```python
from build123d import *

# Parameters (mm, degrees)
BOSS_EXTRUDE1_DEPTH              = 20
SKETCH8_W                        = 42
SKETCH8_H                        = 60
CUT_EXTRUDE1_DEPTH               = 15
CUT_EXTRUDE2_START               = -5
CUT_EXTRUDE2_DEPTH               = 5
SKETCH10_R                       = 36
CUT_EXTRUDE3_DEPTH               = 157.424129235
SKETCH11_R                       = 41
SKETCH11_R_2                     = 36
BOSS_EXTRUDE4_DEPTH              = 5
SKETCH13_W                       = 106.111938503
SKETCH13_H                       = 55
SKETCH13_R                       = 3
BOSS_EXTRUDE9_DEPTH              = 20
BOSS_EXTRUDE13_START             = -5
SKETCH14_R                       = 36
SKETCH14_R_2                     = 33.5
BOSS_EXTRUDE13_DEPTH             = 5
FILLET1_R                        = 10
CUT_EXTRUDE4_DEPTH               = 6
CBORE_FOR_M6_5_SHSS1_D           = 7.1
CBORE_FOR_M6_5_SHSS1_CBORE_D     = 11
CBORE_FOR_M6_5_SHSS1_CBORE_DEPTH = 4.5
CHAMFER5_SIZE                    = 10.579618843
CHAMFER5_SIZE_2                  = 60
CUT_EXTRUDE5_DEPTH               = 1
SKETCH23_W                       = 20
SKETCH23_H                       = 8
CUT_EXTRUDE6_DEPTH               = 34
FILLET5_R                        = 2


with BuildPart() as part:
    # Sketch1 → Boss-Extrude1 (new body)
    with BuildSketch(Plane(origin=(0, 0, 0), x_dir=(1, 0, 0), z_dir=(0, 1, 0))):
        with BuildLine():
            Line((48.082138056, 60.239377577), (47.498980657, -45.87095849))
            ThreePointArc((47.498980657, -45.87095849), (-20.370958489, -112.998980658), (-87.498980658, -45.129041511))
            Line((-87.498980658, -45.129041511), (-86.915823259, 60.981294555))
            ThreePointArc((-86.915823259, 60.981294555), (-19.045884112, 128.109316723), (48.082138056, 60.239377577))
        make_face()
    extrude(amount=BOSS_EXTRUDE1_DEPTH)

    # Sketch8 → Cut-Extrude1 (cut)
    with BuildSketch(Plane.XZ):
        with Locations((-20, -62.5)):
            Rectangle(SKETCH8_W, SKETCH8_H)
    extrude(amount=-CUT_EXTRUDE1_DEPTH, mode=Mode.SUBTRACT)

    # Cut-Extrude2: read off the stored shape, not the designer's step
    # Cut-Extrude2 outline → Cut-Extrude2 (cut)
    with BuildSketch(Plane.XZ.offset(-15).offset(CUT_EXTRUDE2_START)):
        with BuildLine():
            Line((-6.5, -34.5), (-6.5, -90.5))
            ThreePointArc((-6.5, -90.5), (-4.5, -92.5), (-2.5, -90.5))
            Line((-2.5, -90.5), (-2.5, -34.5))
            ThreePointArc((-2.5, -34.5), (-4.5, -32.5), (-6.5, -34.5))
        make_face()
        with BuildLine():
            ThreePointArc((-8, -45), (-20, -33), (-32, -45))
            Line((-32, -45), (-32, -80))
            ThreePointArc((-32, -80), (-20, -92), (-8, -80))
            Line((-8, -80), (-8, -45))
        make_face()
        with BuildLine():
            Line((-37.5, -34.5), (-37.5, -90.5))
            ThreePointArc((-37.5, -90.5), (-35.5, -92.5), (-33.5, -90.5))
            Line((-33.5, -90.5), (-33.5, -34.5))
            ThreePointArc((-33.5, -34.5), (-35.5, -32.5), (-37.5, -34.5))
        make_face()
    extrude(amount=CUT_EXTRUDE2_DEPTH, mode=Mode.SUBTRACT)

    # Sketch10 → Cut-Extrude3 (cut, through all)
    with BuildSketch(Plane.XZ):
        with Locations(Location((-20, 45.5, 0), (0, 0, 270))):
            Circle(SKETCH10_R)
    extrude(amount=-CUT_EXTRUDE3_DEPTH, mode=Mode.SUBTRACT)

    # Sketch11 → Boss-Extrude4 (add)
    with BuildSketch(Plane(origin=(0, 20, 0), x_dir=(1, 0, 0), z_dir=(0, 1, 0))):
        with Locations(Location((-20, -45.5, 0), (0, 0, 270))):
            Circle(SKETCH11_R)
        with Locations(Location((-20, -45.5, 0), (0, 0, 90))):
            Circle(SKETCH11_R_2, mode=Mode.SUBTRACT)
    extrude(amount=BOSS_EXTRUDE4_DEPTH)

    # Sketch13 → Boss-Extrude9 (add)
    with BuildSketch(Plane(origin=(27.749936459, 0, 0.152507111), x_dir=(-0.00549568132488102, 0, 0.999984898629362), z_dir=(-0.999984898629362, 0, -0.00549568132488102))):
        with Locations((-7.446742736, -27.5)):
            Rectangle(SKETCH13_W, SKETCH13_H)
        with Locations((-25.004242736, -10.014310552)):
            Circle(SKETCH13_R, mode=Mode.SUBTRACT)
        with Locations((10.110757264, -10.014310552)):
            Circle(SKETCH13_R, mode=Mode.SUBTRACT)
        with Locations((10.110757264, -39.577999726)):
            Circle(SKETCH13_R, mode=Mode.SUBTRACT)
        with Locations((-25.004242736, -39.514310552)):
            Circle(SKETCH13_R, mode=Mode.SUBTRACT)
    extrude(amount=-BOSS_EXTRUDE9_DEPTH)

    # Sketch14 → Boss-Extrude13 (add)
    with BuildSketch(Plane(origin=(0, 16, 0), x_dir=(1, 0, 0), z_dir=(0, 1, 0)).offset(BOSS_EXTRUDE13_START)):
        with Locations(Location((-20, -45.5, 0), (0, 0, 90))):
            Circle(SKETCH14_R)
        with Locations(Location((-20, -45.5, 0), (0, 0, 270))):
            Circle(SKETCH14_R_2, mode=Mode.SUBTRACT)
    extrude(amount=BOSS_EXTRUDE13_DEPTH)

    # Fillet1
    # the kernel refuses this fillet: 10 mm, written as the material it adds along each edge
    with BuildSketch(Plane(origin=(-20, 11, 45.5), x_dir=(0, 0, -1), z_dir=(1, 0, 0))) as fillet1_piece_1:
        with BuildLine():
            CenterArc((26, -6.614378278), FILLET1_R, 0, 41.409622109)
            Line((36, -6.614378278), (36.2, -6.614378278))
            Line((36.2, -6.614378278), (36.2, 0))
            Line((36.2, 0), (36, 0.2))
            ThreePointArc((36, 0.2), (34.75, 0.2), (33.65, 0.132287566))
            Line((33.65, 0.132287566), (33.5, 0))
        make_face()
    revolve(axis=Axis((-20, 11, 45.5), (0, 1, 0)))

    # Sketch15 → Cut-Extrude4 (cut)
    with BuildSketch(Plane.XZ):
        with BuildLine():
            Line((27.499282685, 45.761044864), (47.498980657, 45.87095849))
            ThreePointArc((47.498980657, 45.87095849), (-20.370958489, 112.998980658), (-87.498980658, 45.129041511))
            Line((-87.498980658, 45.129041511), (-86.915823259, -60.981294555))
            ThreePointArc((-86.915823259, -60.981294555), (-19.045884112, -128.109316723), (48.082138056, -60.239377577))
            Line((48.082138056, -60.239377577), (28.082440084, -60.349291203))
            Line((28.082440084, -60.349291203), (27.499282685, 45.761044864))
        make_face()
    extrude(amount=-CUT_EXTRUDE4_DEPTH, mode=Mode.SUBTRACT)

    # CBORE for M6.5 SHSS1 (through all)
    with Locations(Plane(origin=(27.749936459, 0, 0.152507111), x_dir=(-0.005495681324881029, 0, 0.999984898629362), z_dir=(-0.999984898629362, 0, -0.005495681324881029))):
        with Locations((10.110757264, -39.577999726), (-25.004242736, -39.514310552), (10.110757264, -10.014310552), (-25.004242736, -10.014310552)):
            CounterBoreHole(CBORE_FOR_M6_5_SHSS1_D / 2, CBORE_FOR_M6_5_SHSS1_CBORE_D / 2, CBORE_FOR_M6_5_SHSS1_CBORE_DEPTH)

    # Chamfer5
    # the kernel refuses this chamfer: 60, 10.579618843 mm, written as the material it adds along each edge
    with BuildSketch(Plane(origin=(28.939284552, 6, -216.259264498), x_dir=(-0.9999848986293619, 0, -0.00549568132488103), z_dir=(-0.00549568132488103, 0, 0.999984898629362))) as chamfer5_piece_1_section:
        Polygon((CHAMFER5_SIZE, 0), (0, CHAMFER5_SIZE_2), (0, 0), align=None)
    chamfer5_piece_1 = extrude(amount=417.936594073, mode=Mode.PRIVATE)
    chamfer5_piece_1 = chamfer5_piece_1 - Plane(origin=(27.887351809, -10.014310552, -24.851358027), x_dir=(-0.005495681324881029, 0, 0.999984898629362), z_dir=(-0.999984898629362, 0, -0.005495681324881029)) * Cylinder(5.5, 1076, mode=Mode.PRIVATE)
    chamfer5_piece_1 = chamfer5_piece_1 - Plane(origin=(27.694370959, -10.014310552, 10.263111688), x_dir=(-0.005495681324881029, 0, 0.999984898629362), z_dir=(-0.999984898629362, 0, -0.005495681324881029)) * Cylinder(5.5, 1076, mode=Mode.PRIVATE)
    chamfer5_piece_1 = chamfer5_piece_1 - Plane(origin=(27.887351809, -39.514310552, -24.851358027), x_dir=(-0.005495681324881029, 0, 0.999984898629362), z_dir=(-0.999984898629362, 0, -0.005495681324881029)) * Cylinder(5.5, 1076, mode=Mode.PRIVATE)
    chamfer5_piece_1 = chamfer5_piece_1 - Plane(origin=(27.694370959, -39.577999726, 10.263111688), x_dir=(-0.005495681324881029, 0, 0.999984898629362), z_dir=(-0.999984898629362, 0, -0.005495681324881029)) * Cylinder(5.5, 1076, mode=Mode.PRIVATE)
    chamfer5_piece_1 = split(chamfer5_piece_1, bisect_by=Plane(origin=(27.486315043, -40.618009932, 48.120615135), z_dir=(0.0054121895768273285, 0.17364817766693125, -0.9847928810653225)), keep=Keep.TOP, mode=Mode.PRIVATE)
    chamfer5_piece_1 = split(chamfer5_piece_1, bisect_by=Plane(origin=(28.164666117, 30.853356971, -75.311001495), z_dir=(-0.00541218957682626, 0.17364817766693136, 0.9847928810653225)), keep=Keep.TOP, mode=Mode.PRIVATE)
    add(chamfer5_piece_1)
    with BuildSketch(Plane(origin=(203.992111352, 6, -59.382533108), x_dir=(0.005495681324880034, 0, -0.9999848986293619), z_dir=(-0.999984898629362, 0, -0.005495681324880034))) as chamfer5_piece_2_section:
        Polygon((CHAMFER5_SIZE, 0), (0, CHAMFER5_SIZE_2), (0, 0), align=None)
    chamfer5_piece_2 = extrude(amount=331.824655571, mode=Mode.PRIVATE)
    chamfer5_piece_2 = chamfer5_piece_2 & Plane(origin=(-19.416842601, 6, -60.610336066), x_dir=(-0.999984898629362, 0, -0.005495681324881549), z_dir=(0, -1, 0)) * Cylinder(67.5, 904, mode=Mode.PRIVATE)
    chamfer5_piece_2 = split(chamfer5_piece_2, bisect_by=Plane(origin=(23.126316359, -25.892001157, -60.376528891), z_dir=(0.9847928810653225, 0.1736481776669314, 0.005412189576827241)), keep=Keep.TOP, mode=Mode.PRIVATE)
    add(chamfer5_piece_2)
    with BuildSketch(Plane(origin=(-128.410690611, 6, 44.904200396), x_dir=(-0.005495681324881117, 0, 0.9999848986293619), z_dir=(0.999984898629362, 0, 0.005495681324881118))) as chamfer5_piece_3_section:
        Polygon((CHAMFER5_SIZE, 0), (0, CHAMFER5_SIZE_2), (0, 0), align=None)
    chamfer5_piece_3 = extrude(amount=331.824655571, mode=Mode.PRIVATE)
    chamfer5_piece_3 = chamfer5_piece_3 & Plane(origin=(-20, 6, 45.500000001), x_dir=(0.999984898629362, 0, 0.0054956813248813385), z_dir=(0, -1, 0)) * Cylinder(67.5, 904, mode=Mode.PRIVATE)
    chamfer5_piece_3 = split(chamfer5_piece_3, bisect_by=Plane(origin=(12.537572393, 30.853356971, 45.67881883), z_dir=(0.9847928810653225, 0.1736481776669314, 0.005412189576827241)), keep=Keep.TOP, mode=Mode.PRIVATE)
    add(chamfer5_piece_3)

    # Sketch22 → Cut-Extrude5 (cut)
    with BuildSketch(Plane.XZ.offset(55)):
        Polygon((27.499282685, 45.761044864), (28.082440084, -60.349291203), (48.082138056, -60.239377577), (47.498980657, 45.87095849), align=None)
    extrude(amount=-CUT_EXTRUDE5_DEPTH, mode=Mode.SUBTRACT)

    # Sketch23 → Cut-Extrude6 (cut)
    with BuildSketch(Plane(origin=(47.749634432, 0, 0.262420737), x_dir=(0.005495681324880889, 0, -0.999984898629362), z_dir=(0.999984898629362, 0, 0.005495681324880889))):
        with Locations((49.130161201, -20.643803513)):
            Rectangle(SKETCH23_W, SKETCH23_H)
    extrude(amount=-CUT_EXTRUDE6_DEPTH, mode=Mode.SUBTRACT)

    # Fillet5
    fillet5_edges = [part.edges().sort_by_distance(p)[0] for p in [
        (21.433134302, -16.643803513, -49.01311169),
        (22.083474761, -20.643803513, -39.009386557),
        (22.843728846, -24.643803513, -49.005359395),
        (22.193388387, -20.643803513, -59.009084529),
    ]]
    fillet(fillet5_edges, radius=FILLET5_R)


solid = part.part
```
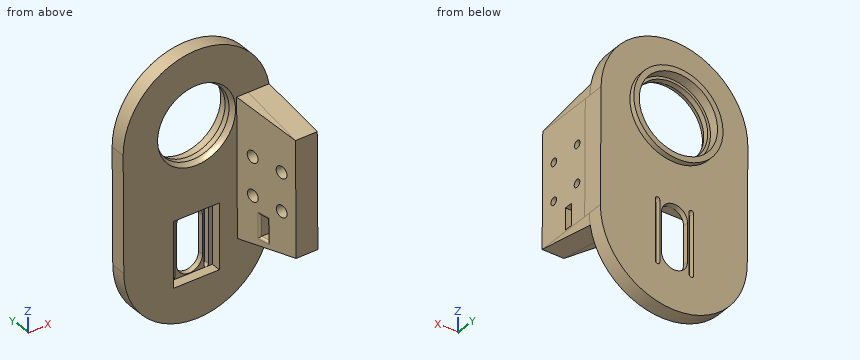
The listing builds one solid part. Answer for the finished solid, in the listing's coordinates (mm). Round coordinates to 2 decimals unless told otherwise and drop trailing zeros. Loops run counter-clockwise (first coordinate to the right, second up) from the corner with the lowest first, then second, coordinate; pieces in that order, holes last. Notation, with made-up numbers: (-26.5, 9.25) - (-11.5, 9.25) arc R9 ccw to (-11.5, 15.25) - close; hole circle Ø3 at (-4, 21). An arc over 180 degrees is marked (long way). Use one line per item in the form item = value. Start each with the question number.
1. The part is cut by section B-B on y = -49. Determine the outline of the cut face in (x, z), then the cut area to 3 significant figures.
2. The part is cut by section D-D on y = -30. Determine the outline of the cut face in (x, z).
3. Consider line 1 (Z direction, x = -20, y = 14); line 2 (X direction, y = 13, z = 45); line 3 (X direction, y = 7, z = -60.5). Determine where each line is inside the solid, lowest interval first. Write a range as [from, to].
4. Given pin 1 Ø4.5 at (x, z) = (-38, -48.5) entering from -Y; pin 2 Ø5.5 at (y, z) = (18, -76.5) entering from -X; pin 3 Ø1.5 at (y, z) = (16.5, -58) entering from +X; pin 4 Ø21.5 at (x, z) = (-26, 34) entering from +Y, each flat-ended and moving along its own axis, determine where each tip first touches the part or whether it passes through.
5. The part is cut by section C-C on z = -67.5. Determine the outline of the cut face in (x, y).
6. The part is cut by section A-A on x = -20. Determine the outline of the cut face in (y, z).
Geometry check:
q1.outline = (26.61, 46.64) - (27.21, -61.24) - (48.08, -61.12) arc R67.5 ccw to (48.08, -60.24) - (47.5, 45.87) arc R67.5 ccw to (47.49, 46.75) - close
q1.area = 2,250 mm^2
q2.outline = (23.24, 49.97) - (23.87, -64.6) - (47.97, -64.47) arc R67.5 ccw to (48.08, -60.24) - (47.5, 45.87) arc R67.5 ccw to (47.34, 50.1) - close
q3.line_1 = [-128.11, -92.5], [-32.5, 12], [79, 113]
q3.line_2 = [-87.5, -53.5], [13.5, 47.5]
q3.line_3 = [-86.92, -41], [1, 48.08]
q4.pin_1 = 15
q4.pin_2 = -85.63
q4.pin_3 = 48.07
q4.pin_4 = through
q5.outline = (-86.56, 6) - (-41, 6) - (-41, 15) - (-37.5, 15) - (-37.5, 20) - (-86.56, 20) - close; (-33.5, 15) - (-32, 15) - (-32, 20) - (-33.5, 20) - close; (-8, 15) - (-6.5, 15) - (-6.5, 20) - (-8, 20) - close; (-2.5, 15) - (1, 15) - (1, 6) - (17.54, 6) - (21.01, -13.67) - (47.73, -12.83) - (47.73, 20) - (-2.5, 20) - close
q6.outline = (6, -128.11) - (20, -128.11) - (20, -92) - (15, -92) - (15, -92.5) - (6, -92.5) - close; (6, -32.5) - (15, -32.5) - (15, -33) - (20, -33) - (20, 4.5) - (25, 4.5) - (25, 9.5) - (16, 9.5) - (16, 12) - (11, 12) arc R10 cw to (6, 9.63) - close; (6, 81.37) arc R10 cw to (11, 79) - (16, 79) - (16, 81.5) - (25, 81.5) - (25, 86.5) - (20, 86.5) - (20, 113) - (6, 113) - close
